Source: CAD feature listing. Evaluate the final solid. Frame: model axes, mm. Face numbers are marked on the shaded views. A direction names the side the tool comes from. Give positions to 0.01 mm unless a question says otherwise; leave off trailing zeros. Loops run counter-clockwise (first coordinate to the right, second up) from the corner with the lowest first, then second, coordinate; pieces in that order, holes last. Notation, with made-up numbers: M -14.75,-8.5 L 9.25,-8.5 A18 ccw 9.25,16.5 Z; hole C 58.25,5.25 d11. An arc over 180 degrees is marked long. Write item = value, one per line.
Autodesk Inventor part; units mm, degrees
ref_plane "YZ Plane" through (0, 0, 0) normal (1, 0, 0) x (0, 1, 0)
ref_plane "XZ Plane" through (0, 0, 0) normal (0, 1, 0) x (-1, 0, 0)
ref_plane "XY Plane" through (0, 0, 0) normal (0, 0, 1) x (1, 0, 0)
ref_plane "Work Plane1" through (0, 0, 0) normal (0, 0, 1) x (1, 0, 0)
sketch "Sketch1" plane through (0, 0, 0) normal (0, 0, 1) x (1, 0, 0)
  circle A0 centre (-10, -25) radius 1.45
  circle A1 centre (-10, 25) radius 1.45
  circle A2 centre (10, 25) radius 1.45
  circle A3 centre (10, -25) radius 1.45
  circle A4 centre (-25, 25) radius 2.325
  circle A5 centre (25, -25) radius 2.325
  circle A6 centre (-25, -25) radius 2.325
  circle A7 centre (25, 25) radius 2.325
  line L0 (28, 30) -> (30, 28)
  line L1 (28, 30) -> (-28, 30)
  line L2 (-30, 28) -> (-28, 30)
  line L3 (-30, 28) -> (-30, -28)
  line L4 (-28, -30) -> (-30, -28)
  line L5 (-28, -30) -> (28, -30)
  line L6 (30, -28) -> (28, -30)
  line L7 (30, -28) -> (30, 28)
  circle A8 centre (-17.5, -17.5) radius 1.95
  circle A9 centre (17.5, 17.5) radius 1.95
  circle A10 centre (17.5, -17.5) radius 1.95
  circle A11 centre (-17.5, 17.5) radius 1.95
  circle A12 centre (0, 0) radius 7.5
  circle A13 centre (-25.33, -75.26) radius 6.15
  circle A14 centre (25, -10) radius 1.45
  circle A15 centre (-25, -10) radius 1.45
  circle A16 centre (-25, 10) radius 1.45
  circle A17 centre (25, 10) radius 1.45
  point P0 (0, 0)
extrude "Extrusion1" add sketch "Sketch1" along normal blind 12 contours L0 L7 L6 L5 L4 L3 L2 L1
sketch "Sketch2" plane through (0, 0, 12) normal (0, 0, 1) x (1, 0, 0)
  circle A0 centre (0, 0) radius 7.5
  circle A1 centre (25, 10) radius 1.45
  circle A2 centre (-25, 10) radius 1.45
  circle A3 centre (-25, -10) radius 1.45
  circle A4 centre (25, -10) radius 1.45
  circle A5 centre (10, -25) radius 1.45
  circle A6 centre (10, 25) radius 1.45
  circle A7 centre (-10, 25) radius 1.45
  circle A8 centre (-10, -25) radius 1.45
  line L0 (-28, -30) -> (28, -30)
  line L1 (28, -30) -> (30, -28)
  line L2 (30, -28) -> (30, 28)
  line L3 (30, 28) -> (28, 30)
  line L4 (28, 30) -> (-28, 30)
  line L5 (30, -28) -> (30, 28)
  line L6 (30, -30) -> (28, -30)
  line L7 (18, -90) -> (30, -90)
  line L8 (30, -90) -> (30, -88) construction
  line L9 (30, 28) -> (30, -28)
  line L10 (30, -30) -> (30, -28)
  line L11 (30, -28) -> (28, -30)
  line L12 (-28, 30) -> (-30, 28)
  line L13 (-30, 28) -> (-30, -28)
  line L14 (-30, -28) -> (-28, -30)
  line L15 (-30, -30) -> (-28, -30)
  line L16 (-18, -90) -> (-30, -90)
  line L17 (-30, -30) -> (-30, -28)
  line L18 (-30, -28) -> (-28, -30)
  line L19 (-28, -30) -> (-30, -30)
  line L20 (28, -30) -> (30, -28)
  line L21 (28, -30) -> (30, -30)
  line L22 (30, -30) -> (30, -28)
  line L23 (30, -28) -> (28, -30)
  circle A9 centre (-17.5, 17.5) radius 1.95
  circle A10 centre (-25, 25) radius 2.325
  circle A11 centre (25, 25) radius 2.325
  circle A12 centre (17.5, 17.5) radius 1.95
  circle A13 centre (17.5, -17.5) radius 1.95
  circle A14 centre (25, -25) radius 2.325
  circle A15 centre (-25, -25) radius 2.325
  line L24 (-18, -90) -> (18, -90)
  line L25 (18, -30) -> (-18, -30)
  line L26 (-50, -90) -> (-32, -90)
  line L27 (50, -90) -> (50, -40) construction
  line L28 (50, -40) -> (30, -40)
  line L29 (-50, -40) -> (-50, -90)
  line L30 (50, -40) -> (98, -40)
  line L31 (100, -40) -> (100, -42)
  line L32 (100, -90) -> (50, -90)
  line L33 (50, -90) -> (50, -40) construction
  line L34 (-30, -40) -> (-30, -30)
  line L35 (-30, -90) -> (-18, -90)
  line L36 (-18, -90) -> (18, -90)
  line L37 (18, -90) -> (30, -90)
  line L38 (30, -90) -> (32, -90)
  line L39 (32, -90) -> (50, -90)
  line L40 (100, -42) -> (100, -90)
  line L41 (98, -40) -> (100, -40)
  line L42 (30, -40) -> (18, -40)
  line L43 (-30, -90) -> (-30, -88) construction
  line L44 (-30, -40) -> (-50, -40)
  line L45 (-30, -88) -> (-30, -40) construction
  line L46 (-32, -90) -> (-30, -90)
  line L47 (18, -40) -> (-18, -40)
  line L48 (-18, -40) -> (-30, -40)
  line L49 (30, -40) -> (30, -30)
  line L50 (30, -88) -> (30, -40) construction
  line L51 (28, -30) -> (18, -30)
  line L52 (-28, -30) -> (-18, -30)
  line L53 (30, -28) -> (30, -30)
  line L54 (30, -28) -> (30, -30)
  line L55 (28, -30) -> (30, -30)
  line L56 (28, -30) -> (30, -28)
  point P0 (0, 0)
  point P1 (-24.2387, -104)
  point P2 (18, -80)
  point P3 (0, -40)
  point P4 (0, -30)
  dimension "d78" = 60
  dimension "d79" = 50
  dimension "d80" = 10
  dimension "d81" = 100
  dimension "d82" = 50
extrude "Extrusion2" add sketch "Sketch2" along normal blind 8
fillet "Fillet1" radius 4 6 edges at (-50, -40, 16) (-50, -90, 16) (100, -90, 16) (100, -40, 16) (30, -40, 16) (-30, -40, 16)
ref_plane "Work Plane2" through (-6, -91, 19) normal (1, 0, 0) x (0, 0, -1)
sketch "Sketch7" plane through (0, 0, 20) normal (0, 0, 1) x (1, 0, 0)
  circle A0 centre (10, -25) radius 1.45
  circle A1 centre (-10, -25) radius 1.45
  circle A2 centre (-25, -10) radius 1.45
  circle A3 centre (-25, 10) radius 1.45
  circle A4 centre (-10, 25) radius 1.45
  circle A5 centre (10, 25) radius 1.45
  circle A6 centre (25, 10) radius 1.45
  circle A7 centre (25, -10) radius 1.45
  circle A8 centre (-25, 25) radius 2.325
  circle A9 centre (25, 25) radius 2.325
  circle A10 centre (25, -25) radius 2.325
  circle A11 centre (-25, -25) radius 2.325
  point P0 (0, 0)
hole "Hole1" at (-25, -10, 20) at (-25, 10, 20) at (-10, 25, 20) at (10, 25, 20) at (25, 10, 20) at (25, -10, 20) at (10, -25, 20) at (-10, -25, 20) at (-25, 25, 20) at (-25, -25, 20) at (25, -25, 20) at (25, 25, 20) direction (0, 0, -1) diameter 3.2 end through all counterbore diameter 8 counterbore depth 10
sketch "Sketch12" plane through (0, 0, 12) normal (0, 0, -1) x (-1, 0, 0)
  line L0 (30.1502, -90.0017) -> (48, -90.0017)
  arc A0 (48, -90.0017) -> (50, -88.0017) centre (48, -88.0017) ccw
  line L1 (50, -70.0017) -> (50, -88.0017)
  arc A1 (50, -41.8579) -> (48, -39.8579) centre (48, -41.8579) ccw
  line L2 (48, -39.8579) -> (30, -39.8579)
  arc A2 (2, -40.0017) -> (0, -42.0017) centre (2, -42.0017) ccw
  line L3 (0, -59.8506) -> (0, -42.0017)
  arc A3 (0, -88.0017) -> (2, -90.0017) centre (2, -88.0017) ccw
  line L4 (9.561, -82.3) -> (40.161, -82.3)
  arc A4 (7.561, -80.3) -> (9.561, -82.3) centre (9.561, -80.3) ccw
  line L5 (7.561, -80.3) -> (7.561, -49.7)
  arc A5 (9.561, -47.7) -> (7.561, -49.7) centre (9.561, -49.7) ccw
  line L6 (40.161, -47.7) -> (9.561, -47.7)
  arc A6 (42.161, -49.7) -> (40.161, -47.7) centre (40.161, -49.7) ccw
  line L7 (42.161, -49.7) -> (42.161, -80.3)
  arc A7 (40.161, -82.3) -> (42.161, -80.3) centre (40.161, -80.3) ccw
  circle A8 centre (46.161, -65) radius 3.89
  circle A9 centre (24.761, -43.7) radius 2.9259
  line L8 (50, -70.0017) -> (50.8263, -70.0017)
  arc A10 (51.3, -70.3417) -> (50.8263, -70.0017) centre (50.8263, -70.5017) ccw
  arc A11 (51.3, -70.3417) -> (53.2596, -71.9417) centre (53.2596, -69.9417) ccw
  line L9 (53.2596, -71.9417) -> (53.4, -71.9417)
  arc A12 (53.4, -71.9417) -> (55.4, -69.9417) centre (53.4, -69.9417) ccw
  line L10 (55.4, -69.9417) -> (55.4, -60.0583)
  arc A13 (55.4, -60.0583) -> (53.4, -58.0583) centre (53.4, -60.0583) ccw
  line L11 (53.4, -58.0583) -> (53.2596, -58.0583)
  arc A14 (53.2596, -58.0583) -> (51.3, -59.6583) centre (53.2596, -60.0583) ccw
  arc A15 (50.8263, -59.9983) -> (51.3, -59.6583) centre (50.8263, -59.4983) ccw
  line L12 (50.8263, -59.9983) -> (50, -59.9983)
  line L13 (50, -41.8579) -> (50, -59.9983)
  line L14 (30, -39.8579) -> (30, -39.1754)
  arc A16 (30.34, -38.7017) -> (30, -39.1754) centre (30.5, -39.1754) ccw
  arc A17 (30.34, -38.7017) -> (31.94, -36.7421) centre (29.94, -36.7421) ccw
  line L15 (31.94, -36.7421) -> (31.94, -36.6017)
  arc A18 (31.94, -36.6017) -> (29.94, -34.6017) centre (29.94, -36.6017) ccw
  line L16 (29.94, -34.6017) -> (20.06, -34.6017)
  arc A19 (20.06, -34.6017) -> (18.06, -36.6017) centre (20.06, -36.6017) ccw
  line L17 (18.06, -36.6017) -> (18.06, -36.7421)
  arc A20 (18.06, -36.7421) -> (19.66, -38.7017) centre (20.06, -36.7421) ccw
  arc A21 (20, -39.1754) -> (19.66, -38.7017) centre (19.5, -39.1754) ccw
  line L18 (20, -39.1754) -> (20, -40.0017)
  line L19 (20, -40.0017) -> (2, -40.0017)
  line L20 (19.8489, -90.0017) -> (19.8491, -89.2759)
  arc A22 (19.8491, -89.2759) -> (19.6194, -88.9515) centre (19.5001, -89.2795) ccw
  arc A23 (17.9053, -86.8424) -> (19.6194, -88.9515) centre (20.06, -86.8424) ccw
  line L21 (17.9053, -86.8424) -> (17.9053, -86.7026)
  arc A24 (20.0566, -84.5515) -> (17.9053, -86.7026) centre (20.0565, -86.7026) ccw
  line L22 (20.0566, -84.5515) -> (29.94, -84.552)
  arc A25 (32.09, -86.7021) -> (29.94, -84.552) centre (29.94, -86.702) ccw
  line L23 (32.09, -86.7021) -> (32.09, -86.8424)
  arc A26 (30.38, -88.9468) -> (32.09, -86.8424) centre (29.9401, -86.8423) ccw
  arc A27 (30.38, -88.9468) -> (30.1502, -89.2756) centre (30.5004, -89.2756) ccw
  line L24 (30.1502, -89.2756) -> (30.1502, -90.0017)
  line L25 (0, -59.8506) -> (0.7258, -59.8508)
  arc A28 (0.7258, -59.8508) -> (1.0502, -59.6211) centre (0.7222, -59.5018) ccw
  arc A29 (3.1593, -57.907) -> (1.0502, -59.6211) centre (3.1593, -60.0617) ccw
  line L26 (3.1593, -57.907) -> (3.2991, -57.907)
  arc A30 (5.4502, -60.0583) -> (3.2991, -57.907) centre (3.2991, -60.0582) ccw
  line L27 (5.4502, -60.0583) -> (5.4497, -69.9417)
  arc A31 (3.2996, -72.0917) -> (5.4497, -69.9417) centre (3.2997, -69.9417) ccw
  line L28 (3.2996, -72.0917) -> (3.1593, -72.0917)
  arc A32 (1.0549, -70.3817) -> (3.1593, -72.0917) centre (3.1594, -69.9418) ccw
  arc A33 (1.0549, -70.3817) -> (0.7261, -70.1519) centre (0.7261, -70.5021) ccw
  line L29 (0.7261, -70.1519) -> (0, -70.152)
  line L30 (0, -88.0017) -> (0, -70.152)
  line L31 (2, -90.0017) -> (19.8489, -90.0017)
  line L32 (50, -44) -> (50, -86)
  line L33 (-0.1817, -64.8173) -> (24.3267, -108.886) construction
  line L34 (-100, -86) -> (-100, -44)
  line L35 (50, -44) -> (50, -86)
  point P0 (24.211, -65)
  point P1 (50, -65)
  point P2 (55.4, -65)
  point P3 (42.161, -65)
  point P4 (50, -65)
  point P5 (5.45, -65)
  point P6 (50, -65)
  point P7 (7.561, -65)
  point P8 (50, -65)
  point P9 (50, -65)
  dimension "d106" = 7.78
  dimension "d107" = 4
  dimension "d108" = 21.4
  dimension "d109" = 4
hole "Hole2" at (-46.161, -65, 12) at (-24.761, -43.7, 12) direction (0, 0, 1) diameter 3.2 end through all
pattern_linear "Rectangular Pattern1" count 3 spacing 50 along (1, 0, 0) of "Hole2"
sketch "Sketch15" plane through (0, 0, 12) normal (0, 0, -1) x (-1, 0, 0)
  line L0 (50, -40) -> (0, -40)
  line L1 (-100, -40) -> (-100, -90)
  line L2 (-100, -90) -> (-50, -90)
  line L3 (50, -90) -> (50, -40)
  line L4 (46, -90) -> (-96, -90)
  line L5 (-50, -40) -> (-50, -90)
  line L6 (50, -44) -> (50, -86)
  arc A0 (50, -44) -> (46, -40) centre (46, -44) ccw
  line L7 (34, -40) -> (46, -40)
  arc A1 (30, -36) -> (34, -40) centre (34, -36) ccw
  line L8 (30, -28) -> (30, -36)
  arc A2 (46, -90) -> (50, -86) centre (46, -86) ccw
  line L9 (46, -90) -> (-96, -90)
  arc A3 (-100, -86) -> (-96, -90) centre (-96, -86) ccw
  line L10 (-100, -86) -> (-100, -44)
  arc A4 (-96, -40) -> (-100, -44) centre (-96, -44) ccw
  line L11 (-96, -40) -> (-34, -40)
  arc A5 (-34, -40) -> (-30, -36) centre (-34, -36) ccw
  line L12 (-30, -36) -> (-30, -28)
  line L13 (0, -40) -> (0, -90)
  line L14 (42.3, -47.7) -> (7.7, -47.7)
  line L15 (7.7, -47.7) -> (7.7, -82.3)
  line L16 (7.7, -82.3) -> (42.3, -82.3)
  line L17 (42.3, -82.3) -> (42.3, -47.7)
  line L18 (-7.7, -47.7) -> (-42.3, -47.7)
  line L19 (-42.3, -47.7) -> (-42.3, -82.3)
  line L20 (-42.3, -82.3) -> (-7.7, -82.3)
  line L21 (-7.7, -82.3) -> (-7.7, -47.7)
  line L22 (-57.7, -47.7) -> (-92.3, -47.7)
  line L23 (-92.3, -47.7) -> (-92.3, -82.3)
  line L24 (-92.3, -82.3) -> (-57.7, -82.3)
  line L25 (-57.7, -82.3) -> (-57.7, -47.7)
  line L26 (0, -90) -> (50, -90)
  line L27 (-50, -90) -> (0, -90)
  line L28 (-50, -40) -> (-100, -40)
  line L29 (0, -40) -> (-50, -40)
  point P0 (0, 0)
  point P1 (0, -65)
  point P2 (42.3, -65)
  point P3 (50, -65)
  point P4 (-7.7, -65)
  point P5 (50, -65)
  point P6 (50, -65)
  point P7 (-57.7, -65)
  point P8 (25, -82.3)
  point P9 (25, -90)
  point P10 (-25, -82.3)
  point P11 (-25, -90)
  point P12 (-75, -82.3)
  point P13 (-75, -90)
  dimension "d116" = 50
  dimension "d117" = 50
  dimension "d118" = 50
  dimension "d119" = 34.6
  dimension "d120" = 34.6
  dimension "d121" = 34.6
  dimension "d122" = 34.6
  dimension "d123" = 34.6
  dimension "d124" = 34.6
extrude "Extrusion10" cut sketch "Sketch15" against normal blind 10 contours L17 L16 L15 L14 | L21 L20 L19 L18 | L25 L24 L23 L22
fillet "Fillet2" radius 2 12 edges at (-42.3, -82.3, 16) (-42.3, -47.7, 16) (-7.7, -47.7, 16) (42.3, -47.7, 16) (-7.7, -82.3, 16) (7.7, -47.7, 16) (7.7, -82.3, 16) (57.7, -82.3, 16) (42.3, -82.3, 16) (92.3, -82.3, 16) (57.7, -47.7, 16) (92.3, -47.7, 16)
ref_plane "Work Plane3" through (-46, -65, 12) normal (0, -1, 0) x (1, 0, 0)
mirror "Mirror2" about plane through (-46, -65, 12) normal (0, -1, 0) of "Hole2", "Rectangular Pattern1"
properties part number "30_XY_Sample_arm_UC2_Adapter_v3"
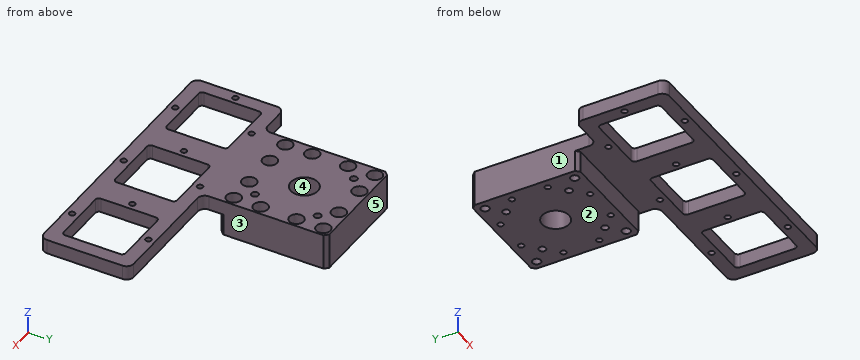
1. Pull-direction query (Y, two-part tool) for the marked faces 3, 4 and 5; classes: +Y half, -Y half, draft (parallel to the pull), parting line (faces both ways), or undercut.
Derived:
face_3 = draft
face_4 = undercut
face_5 = +Y half
2. First-contact query: pin 1 Ø12 at (x, y) = (77, -42.5) entering from -Z; pin 2 Ø10 at (x, z) = (56.5, 8) entering from +Y; pin 3 Ø1.5 at (y, z) = (-27.5, 10) entering from -X. Flat tips, straight axial feed; report the tip coordinate or a pass-through.
Derived:
pin_1 = 12
pin_2 = -40
pin_3 = -30
3. Cut plane C-C, the plane x = 72. Return the cut outline in (y, z), then the cut area to 3 significant figures.
Derived:
outline = M -90,12 L -82.3,12 L -82.3,20 L -90,20 Z; M -47.7,12 L -40,12 L -40,20 L -47.7,20 Z
area = 123 mm²
4. Cut plane A-A, the plane z = 6. Count the separate pieces of the cut face and the enclosed holes in it, then the cut area to 3 significant figures.
Derived:
separate_pieces = 1
enclosed_holes = 17
area = 3,240 mm²
5. Reachability of the marked faces 1 and 2 from +Z, -Z, +X, -X, +Y, -Y: full face, straight path, thin tool, end or side. Return the list, or none.
Derived:
face_1 = +Z, -Z, -X, +Y
face_2 = -Z, +X, -X, +Y, -Y
6. Material intervals for probe 1 along X at (y, z) = (-52, 18); probe 2 along Y at (x, z) = (-25, 11); probe 3 along Y at (x, z) = (25, 5.25) (3 decimals), sorted ascending. Write a range as from..to.
Derived:
probe_1 = -50..-42.3, -7.7..7.7, 42.3..57.7, 92.3..100
probe_2 = -30..-29, -21..-14, -6..6, 14..21, 29..30
probe_3 = -30..-27.325, -22.675..-11.6, -8.4..8.4, 11.6..22.675, 27.325..30
7. Cut plane D-D, the plane y = 17.5. Return the cut outline in (x, z).
Derived:
outline = M -30,0 L -19.45,0 L -19.45,20 L -30,20 Z; M -15.55,0 L 15.55,0 L 15.55,20 L -15.55,20 Z; M 19.45,0 L 30,0 L 30,20 L 19.45,20 Z
8. Cut plane B-B, the plane y = 0. Return the cut outline in (x, z), then the cut area to 3 significant figures.
Derived:
outline = M -30,0 L -7.5,0 L -7.5,20 L -30,20 Z; M 7.5,0 L 30,0 L 30,20 L 7.5,20 Z
area = 900 mm²
